Can you work these out from the model? Positions are in its coordinate system, mm. A direction names the side the tool comes from. Coordinates: 2 decimals unless noted, no trailing zeros. Order: outer loops, then holes, each group sorted by start corner. A loop starts at its lowest first (then second) coordinate and runs counter-clockwise, first axis right, second up. Notation, with made-up numbers: (-1, -13) -> (11, -13) arc R14 cw to (11, 7) -> close; hole circle Ø9 at (8, -25). An arc over 180 degrees is marked (long way). Write item = value, one per line.
```python
from build123d import *

# Parameters (mm, degrees)
F0_R     = 24.15767
F1_DEPTH = 38.1
F2_COUNT = 24


with BuildPart() as f1:
    # F0 (on Right) → F1 (new body, symmetric)
    with BuildSketch(Plane.YZ):
        with BuildLine():
            ThreePointArc((-1.84246, 26.538285), (-18.147477, -19.451076), (26.602166, 0))
            ThreePointArc((26.602166, 0), (19.369196, 18.234843), (1.603488, 26.553796))
            ThreePointArc((1.603488, 26.553796), (-0.119738, 26.601897), (-1.84246, 26.538285))
        make_face()
        Circle(F0_R, mode=Mode.SUBTRACT)
        with BuildLine():
            ThreePointArc((-1.84246, 26.538285), (-0.119738, 26.601897), (1.603488, 26.553796))
            Line((1.603488, 26.553796), (1.603488, 31.000791))
            Line((1.603488, 31.000791), (-1.84246, 31.000791))
            Line((-1.84246, 31.000791), (-1.84246, 26.538285))
        make_face()
    extrude(amount=F1_DEPTH, both=True)

    # F2: F1 ×24 about axis
    f2_axis = Axis((0, 0, 0), (1, 0, 0))


with BuildPart() as f1_1:
    add(f1.part)
    for i in range(1, F2_COUNT):
        add(f1.part.rotate(f2_axis, i * 360 / F2_COUNT))


solid = f1_1.part
```
Item 1: If I drill on probe 1 along Y at (x, z) = (-9, 0); probe 2 along Y at (x, z) = (-7, -21), over which ranges is the centre line in solid material (lowest first)?
A:
probe_1 = -31 to -24.16, 24.16 to 31
probe_2 = -22.84 to -18.39, -16.33 to -11.94, 11.94 to 16.33, 18.73 to 22.84
Item 2: If we mould it in two halves opening along Y, with no side actions, what happens to faces 5 (the flat face through (0.533, 24.021, 15.996)), 6 (the cylindrical face through (0.533, -3.378, -26.387)), 7 (the flat face through (1, -29, 1.603)), 8 (the cylindrical face through (0.533, -26.387, 3.378))? For each: pulls with the +Y half, pulls with the -Y half, needs draft (parallel to the pull), parting line crosses it, or undercut.
A:
face_5 = undercut
face_6 = undercut
face_7 = needs draft
face_8 = pulls with the -Y half
Item 3: For faces 1 (the flat face through (0.533, 28.296, -5.675)), 2 (the flat face through (0.5, 9, 27.4)), 3 (the flat face through (0.533, -12.984, 25.697)), 4 (the flat face through (1, -1.603, -29)), which set-ups out of +Z, -Z, +X, -X, +Y, -Y let a thin tool reach every point of the face, with its end or its side?
A:
face_1 = +X, -X, +Y
face_2 = +X, -X
face_3 = +Z, +X, -X
face_4 = -Z, +X, -X
Item 4: I'm going to push flat-ended pins straight in: P1, Ø1.5, axis at x = 16, z = 8.5, coming from the -Y side; P2, Ø3.5, axis at x = -11, y = -28, coming from the -Z side; P3, Ø5, axis at x = -17.5, z = 28, coming from the +Y side. Where does each tip first touch, or does it pass through?
A:
P1 = -30.02
P2 = -16.54
P3 = 16.89
Item 5: I want a section at A-A, the plane y = 0. Please give me the cut outline in (x, z), plus the area to 3 significant figures.
A:
outline = (-38.1, -31) -> (38.1, -31) -> (38.1, -24.16) -> (-38.1, -24.16) -> close; (-38.1, 24.16) -> (38.1, 24.16) -> (38.1, 31) -> (-38.1, 31) -> close
area = 1,040 mm2
